The model under review builds one solid part; all positions refer to its coordinate system, in mm. A direction names the side the tool comes from. Round coordinates to 2 decimals unless told otherwise and drop trailing zeros. Loops run counter-clockwise (first coordinate to the right, second up) from the corner with the lowest first, then second, coordinate; pieces in that order, holes last. Notation, with made-up numbers: M 85.5,68.5 L 111.5,68.5 A12 ccw 111.5,74.5 Z; hole C -18.5,60.25 d8. An arc over 180 degrees is marked long. Return JSON: item names as keys, results as strings. Group by question number.
Q1. To check wall thickness, follow line 1 along X through (y, z) = (-6.5, -27); line 2 along Z through (x, y) = (-17, -4); line 3 along Z through (x, y) = (-22, -2.75). State the ranges of each line that lie inside material, in increasing order.
Q2. Draft analysis for pull direction X (two halves, no side actions). For faces 1 (the face through (-18, -11.78, -7)), 2 (the face through (23, -11.78, -6)), 3 (the face through (43, -24, -57)), 4 (the face through (-1, 0, -70)), state which applies: pulls with the +X half, pulls with the -X half, needs draft (parallel to the pull), parting line crosses it, or undercut.
Q3. For faces 5 (the face through (-45, -12, -57)), 6 (the face through (22, -11.78, -26)), 7 (the face through (17.03, -23.03, -21.22)), list the 3-axis set-ups (+Z, -Z, +X, -X, +Y, -Y) from which the entire face can be reached by the end or side of a thin tool; tool diameter is ignored.
Q4. Consider section A-A (y = -9.5). State the section outline as (x, z) points (3 decimals).
Q5. Clearance check with flat-ended pins moving along their axes: pin 1 Ø6.5 at (x, z) = (-20.075, -5.855) entering from +Y; pin 2 Ø3 at (x, y) = (3.5, -3) entering from +Z; pin 3 Ø1.7 at (y, z) = (-4, -12.5) entering from +X. State where each tip first meets the part, or that it passes through.
from build123d import *

# Parameters (mm, degrees)
F1_DEPTH       = 25
F3_DEPTH       = 5.78
F4_DEPTH       = 11.78
F5_R           = 5
F6_R           = 5
F8_D           = 4.4
F8_CBORE_D     = 8.25
F8_CBORE_DEPTH = 4


with BuildPart() as f1:
    # F0 (on Front) → F1 (new body)
    with BuildSketch(Plane.XZ):
        with BuildLine():
            Line((40, 10), (-40, 10))
            ThreePointArc((-40, 10), (-43.5355339059, 8.5355339059), (-45, 5))
            Line((-45, 5), (-45, -119.86))
            ThreePointArc((-45, -119.86), (-43.5355339059, -123.3955339059), (-40, -124.86))
            Line((-40, -124.86), (40, -124.86))
            ThreePointArc((40, -124.86), (43.5355339059, -123.3955339059), (45, -119.86))
            Line((45, -119.86), (45, 5))
            ThreePointArc((45, 5), (43.5355339059, 8.5355339059), (40, 10))
        make_face()
    extrude(amount=F1_DEPTH)

    # F2 (on Front) → F3 (cut)
    with BuildSketch(Plane.XZ):
        Polygon((24.46, 0), (-24.46, 0), (-24.46, -17.86), (-26.955, -17.86), (-26.955, -29.86), (26.955, -29.86), (26.955, -17.86), (24.46, -17.86), align=None)
        with BuildLine():
            ThreePointArc((-20.075, -9.605), (-22.7266504294, -3.2033495706), (-16.325, -5.855))
            Line((-16.325, -5.855), (16.325, -5.855))
            ThreePointArc((16.325, -5.855), (20.075, -2.105), (23.825, -5.855))
            ThreePointArc((23.825, -5.855), (22.7266504294, -8.5066504294), (20.075, -9.605))
            Line((20.075, -9.605), (20.075, -20.255))
            ThreePointArc((20.075, -20.255), (22.7266504294, -21.3533495706), (23.825, -24.005))
            ThreePointArc((23.825, -24.005), (20.075, -27.755), (16.325, -24.005))
            Line((16.325, -24.005), (-16.325, -24.005))
            ThreePointArc((-16.325, -24.005), (-22.7266504294, -26.6566504294), (-20.075, -20.255))
            Line((-20.075, -20.255), (-20.075, -9.605))
        make_face(mode=Mode.SUBTRACT)
        with BuildLine():
            Line((16.325, -5.855), (-16.325, -5.855))
            ThreePointArc((-16.325, -5.855), (-17.4233495706, -8.5066504294), (-20.075, -9.605))
            Line((-20.075, -9.605), (-20.075, -20.255))
            ThreePointArc((-20.075, -20.255), (-17.4233495706, -21.3533495706), (-16.325, -24.005))
            Line((-16.325, -24.005), (16.325, -24.005))
            ThreePointArc((16.325, -24.005), (17.4233495706, -21.3533495706), (20.075, -20.255))
            Line((20.075, -20.255), (20.075, -9.605))
            ThreePointArc((20.075, -9.605), (17.4233495706, -8.5066504294), (16.325, -5.855))
        make_face()
    extrude(amount=F3_DEPTH, mode=Mode.SUBTRACT)

    # F2 (on Front) → F4 (cut, through all)
    with BuildSketch(Plane.XZ):
        with BuildLine():
            Line((-16.325, -5.855), (-18.45, -5.855))
            ThreePointArc((-18.45, -5.855), (-18.9259514806, -7.0040485194), (-20.075, -7.48))
            Line((-20.075, -7.48), (-20.075, -9.605))
            ThreePointArc((-20.075, -9.605), (-17.4233495706, -8.5066504294), (-16.325, -5.855))
        make_face()
        with BuildLine():
            Line((-18.45, -5.855), (-20.075, -5.855))
            Line((-20.075, -5.855), (-20.075, -7.48))
            ThreePointArc((-20.075, -7.48), (-18.9259514806, -7.0040485194), (-18.45, -5.855))
        make_face()
        with BuildLine():
            Line((-20.075, -7.48), (-20.075, -5.855))
            Line((-20.075, -5.855), (-18.45, -5.855))
            ThreePointArc((-18.45, -5.855), (-21.2240485194, -4.7059514806), (-20.075, -7.48))
        make_face()
        with BuildLine():
            ThreePointArc((-20.075, -7.48), (-21.2240485194, -4.7059514806), (-18.45, -5.855))
            Line((-18.45, -5.855), (-16.325, -5.855))
            ThreePointArc((-16.325, -5.855), (-22.7266504294, -3.2033495706), (-20.075, -9.605))
            Line((-20.075, -9.605), (-20.075, -7.48))
        make_face()
        with BuildLine():
            ThreePointArc((-16.325, -24.005), (-17.4233495706, -21.3533495706), (-20.075, -20.255))
            Line((-20.075, -20.255), (-20.075, -22.38))
            ThreePointArc((-20.075, -22.38), (-18.9259514806, -22.8559514806), (-18.45, -24.005))
            Line((-18.45, -24.005), (-16.325, -24.005))
        make_face()
        with BuildLine():
            ThreePointArc((-18.45, -24.005), (-18.9259514806, -22.8559514806), (-20.075, -22.38))
            Line((-20.075, -22.38), (-20.075, -24.005))
            Line((-20.075, -24.005), (-18.45, -24.005))
        make_face()
        with BuildLine():
            Line((-20.075, -22.38), (-20.075, -20.255))
            ThreePointArc((-20.075, -20.255), (-22.7266504294, -26.6566504294), (-16.325, -24.005))
            Line((-16.325, -24.005), (-18.45, -24.005))
            ThreePointArc((-18.45, -24.005), (-21.2240485194, -25.1540485194), (-20.075, -22.38))
        make_face()
        with BuildLine():
            Line((-20.075, -24.005), (-20.075, -22.38))
            ThreePointArc((-20.075, -22.38), (-21.2240485194, -25.1540485194), (-18.45, -24.005))
            Line((-18.45, -24.005), (-20.075, -24.005))
        make_face()
        with BuildLine():
            Line((18.45, -5.855), (16.325, -5.855))
            ThreePointArc((16.325, -5.855), (17.4233495706, -8.5066504294), (20.075, -9.605))
            Line((20.075, -9.605), (20.075, -7.48))
            ThreePointArc((20.075, -7.48), (18.9259514806, -7.0040485194), (18.45, -5.855))
        make_face()
        with BuildLine():
            Line((20.075, -5.855), (18.45, -5.855))
            ThreePointArc((18.45, -5.855), (18.9259514806, -7.0040485194), (20.075, -7.48))
            Line((20.075, -7.48), (20.075, -5.855))
        make_face()
        with BuildLine():
            ThreePointArc((23.825, -5.855), (20.075, -2.105), (16.325, -5.855))
            Line((16.325, -5.855), (18.45, -5.855))
            ThreePointArc((18.45, -5.855), (20.075, -4.23), (21.7, -5.855))
            ThreePointArc((21.7, -5.855), (21.2240485194, -7.0040485194), (20.075, -7.48))
            Line((20.075, -7.48), (20.075, -9.605))
            ThreePointArc((20.075, -9.605), (22.7266504294, -8.5066504294), (23.825, -5.855))
        make_face()
        with BuildLine():
            ThreePointArc((21.7, -5.855), (20.075, -4.23), (18.45, -5.855))
            Line((18.45, -5.855), (20.075, -5.855))
            Line((20.075, -5.855), (20.075, -7.48))
            ThreePointArc((20.075, -7.48), (21.2240485194, -7.0040485194), (21.7, -5.855))
        make_face()
        with BuildLine():
            Line((20.075, -22.38), (20.075, -20.255))
            ThreePointArc((20.075, -20.255), (17.4233495706, -21.3533495706), (16.325, -24.005))
            Line((16.325, -24.005), (18.45, -24.005))
            ThreePointArc((18.45, -24.005), (18.9259514806, -22.8559514806), (20.075, -22.38))
        make_face()
        with BuildLine():
            Line((20.075, -24.005), (20.075, -22.38))
            ThreePointArc((20.075, -22.38), (18.9259514806, -22.8559514806), (18.45, -24.005))
            Line((18.45, -24.005), (20.075, -24.005))
        make_face()
        with BuildLine():
            ThreePointArc((21.7, -24.005), (21.2240485194, -22.8559514806), (20.075, -22.38))
            Line((20.075, -22.38), (20.075, -24.005))
            Line((20.075, -24.005), (18.45, -24.005))
            ThreePointArc((18.45, -24.005), (20.075, -25.63), (21.7, -24.005))
        make_face()
        with BuildLine():
            ThreePointArc((23.825, -24.005), (22.7266504294, -21.3533495706), (20.075, -20.255))
            Line((20.075, -20.255), (20.075, -22.38))
            ThreePointArc((20.075, -22.38), (21.2240485194, -22.8559514806), (21.7, -24.005))
            ThreePointArc((21.7, -24.005), (20.075, -25.63), (18.45, -24.005))
            Line((18.45, -24.005), (16.325, -24.005))
            ThreePointArc((16.325, -24.005), (20.075, -27.755), (23.825, -24.005))
        make_face()
    extrude(amount=F4_DEPTH, mode=Mode.SUBTRACT)

    # F5
    f5_edges = [f1.edges().sort_by_distance(p)[0] for p in [
        (0, 0, -124.86),
        (-43.535534, 0, -123.395534),
        (43.535534, 0, -123.395534),
        (45, 0, -57.43),
        (-45, 0, -57.43),
        (0, 0, 10),
        (-43.535534, 0, 8.535534),
        (43.535534, 0, 8.535534),
    ]]
    fillet(f5_edges, radius=F5_R)

    # F6
    f6_edges = [f1.edges().sort_by_distance(p)[0] for p in [
        (0, -25, -124.86),
    ]]
    fillet(f6_edges, radius=F6_R)

    # F8 (through all)
    with Locations(Plane.XZ.offset(25)):
        with Locations((-20.075, -24.005), (-20.075, -5.855), (20.075, -5.855), (20.075, -24.005)):
            CounterBoreHole(F8_D / 2, F8_CBORE_D / 2, F8_CBORE_DEPTH)


solid = f1.part
Values:
{
 "1": {"line 1": "x = -45 to -22.33, -17.82 to 17.82, 22.33 to 45", "line 2": "z = -124.76 to -29.86, 0 to 9.9", "line 3": "z = -124.33 to -29.86, 0 to 9.47"},
 "2": {"face 1": "undercut", "face 2": "undercut", "face 3": "pulls with the +X half", "face 4": "needs draft"},
 "3": {"face 5": "+Z, -Z, -X, +Y, -Y", "face 6": "+Y", "face 7": "-Y"},
 "4": {"outline": "M -45,-119.86 A5 ccw -40,-124.86 L 40,-124.86 A5 ccw 45,-119.86 L 45,5 A5 ccw 40,10 L -40,10 A5 ccw -45,5 Z; hole C -20.075,-24.005 d7.5; hole C -20.075,-5.855 d7.5; hole C 20.075,-24.005 d7.5; hole C 20.075,-5.855 d7.5"},
 "5": {"pin 1": "stops at y = -11.78", "pin 2": "stops at z = 9.97", "pin 3": "stops at x = 45"}
}
